Answer from the drawing. Dimensions are ordinates in mm from the lowest x, y and z of the part. A direction names the side the tool comes from. Give positions to 0.01 mm unless a question says otherwise; leave off trailing zeros. Write each loop counter-clockwise with the first axis right and the second up, starting at its lowest first coordinate (ties: lowest second). Pieces come first, ordered by that corner, then holes. Notation, with made-up numbers: M 60,22 L 73,22 A28 ccw 73,49 Z; hole C -14.5,28.25 d8. An arc over 180 degrees is marked long. Answer as a JSON object with one key per item and string values.
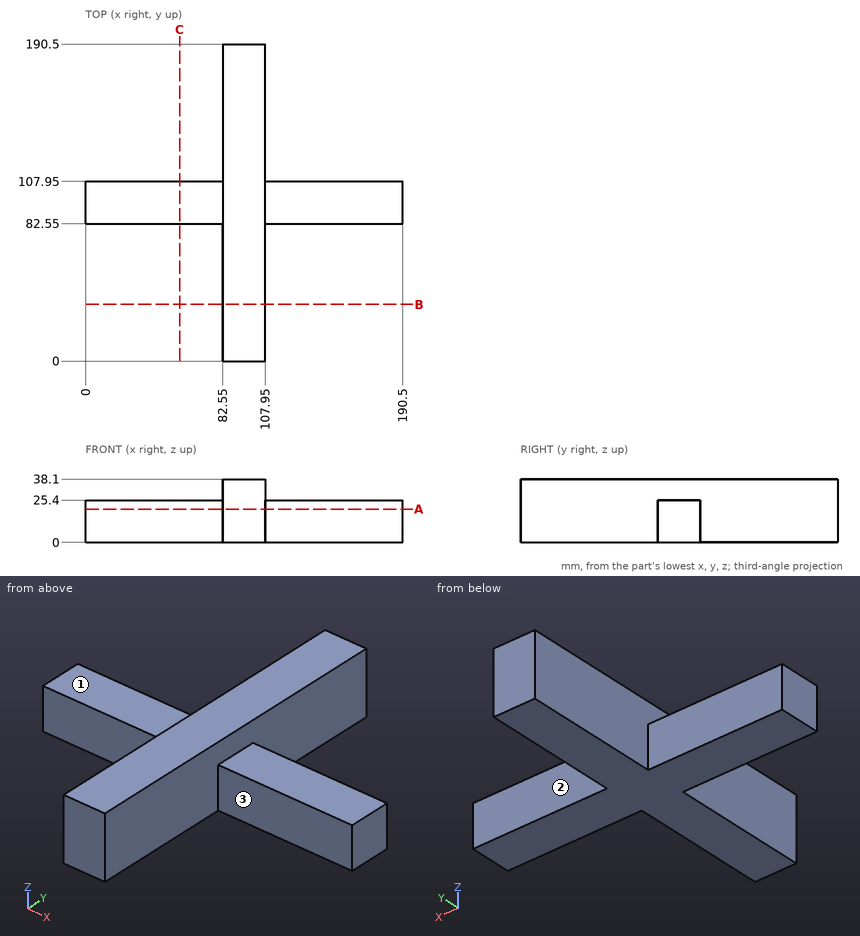
1. A cutting plane is placed at B-B, the plane y = 34. Give the vertices of the cut face in (x, z).
Verdict:
{"outline": "M 82.55,0 L 107.95,0 L 107.95,38.1 L 82.55,38.1 Z"}
2. Consider line 1 along X through (y, z) = (19, 23); line 2 along Z through (x, y) = (70, 84). Determine where each line is inside the solid, lowest interval first.
Verdict:
{"line 1": "x = 82.55 to 107.95", "line 2": "z = 0 to 25.4"}
3. Flat-ended cylindrical pins translate along their axes: pin 1 (12.5 mm diameter, centred on x = 137.5, z = 16.5, fed in from +Y); pin 2 (12.5 mm diameter, centred on x = 44, z = 9, fed in from -Y); pin 3 (12 mm diameter, centred on y = 154, z = 4.5, fed in from +X). Find the tip coordinate at first contact, or state that the pin passes through.
Verdict:
{"pin 1": "stops at y = 107.95", "pin 2": "stops at y = 82.55", "pin 3": "stops at x = 107.95"}
4. For the marked faces 1, 2 and 3, determine the directions among +Z, -Z, +X, -X, +Y, -Y from which every point of the face is accessible in a straight line to the end or side of a thin tool.
Verdict:
{"face 1": "+Z, -X, +Y, -Y", "face 2": "+Z, -Z, +X, +Y", "face 3": "+Z, -Z, +X, -Y"}
5. A cutting plane is placed at C-C, the plane x = 56.5. Give the vertices of the cut face in (y, z), plus the area to 3 significant figures.
Verdict:
{"outline": "M 82.55,0 L 107.95,0 L 107.95,25.4 L 82.55,25.4 Z", "area": "645 mm2"}
6. A cutting plane is placed at A-A, the plane z = 20. Give the vertices of the cut face in (x, y), plus the area to 3 significant figures.
Verdict:
{"outline": "M 0,82.55 L 82.55,82.55 L 82.55,0 L 107.95,0 L 107.95,82.55 L 190.5,82.55 L 190.5,107.95 L 107.95,107.95 L 107.95,190.5 L 82.55,190.5 L 82.55,107.95 L 0,107.95 Z", "area": "9,030 mm2"}
